Build history of the part. All positions in model axes, mm. Coordinates: 2 decimals unless noted, no trailing zeros. Order: outer loops, then holes, each group sorted by start corner. A loop starts at its lowest first (then second) coordinate and runs counter-clockwise, first axis right, second up. Notation, with made-up numbers: (51.5, 21.25) - (79.5, 21.25) arc R28 cw to (79.5, 39.25) - close; hole circle Ø1 at (5, 72). An arc over 180 degrees is marked (long way). Answer as CSV lines item,"result". Start each with the question number.
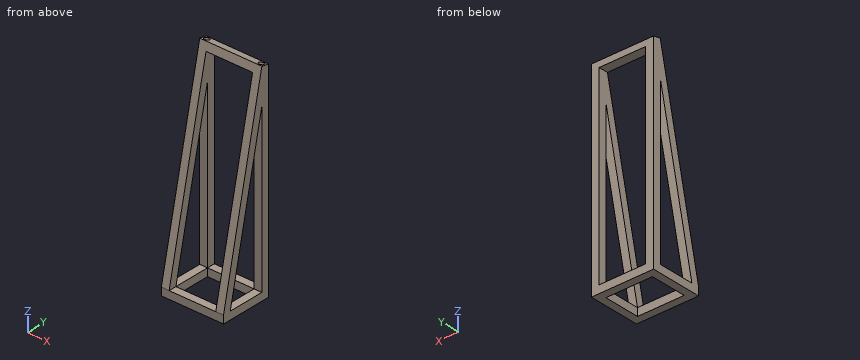
from build123d import *

# Parameters (mm, degrees)
F1_DEPTH = 30.48
F2_W     = 22.86
F2_H     = 93.98
F3_DEPTH = 25.4
F4_W     = 22.86
F4_H     = 17.78
F5_DEPTH = 25.4
F7_DEPTH = 50.8
F8_R     = 1.27
F9_DEPTH = 25.4


with BuildPart() as f1:
    # F0 (on Right) → F1 (new body)
    with BuildSketch(Plane.YZ):
        Polygon((-30.7647287846, 64.6939707769), (-52.3547287846, -33.0960292231), (-48.5447287846, -33.0960292231), (-30.7647287846, 47.4369119534), align=None)
        Polygon((-52.3547287846, -33.0960292231), (-52.3547287846, -36.9060292231), (-26.9547287846, -36.9060292231), (-26.9547287846, -33.0960292231), (-30.7647287846, -33.0960292231), (-48.5447287846, -33.0960292231), align=None)
        Polygon((-30.7647287846, -33.0960292231), (-26.9547287846, -33.0960292231), (-26.9547287846, 64.6939707769), (-30.7647287846, 47.4369119534), align=None)
        Polygon((-26.9547287846, 64.6939707769), (-30.7647287846, 64.6939707769), (-30.7647287846, 47.4369119534), align=None)
    extrude(amount=F1_DEPTH)

    # F2 (on face) → F3 (cut)
    with BuildSketch(Plane(origin=(0, -26.9547287846, 0), x_dir=(-1, 0, 0), z_dir=(0, 1, 0))):
        with Locations((-15.24, 13.8939707769)):
            Rectangle(F2_W, F2_H)
    extrude(amount=-F3_DEPTH, mode=Mode.SUBTRACT)

    # F4 (on face) → F5 (cut)
    with BuildSketch(Plane.XY.offset(-33.0960292231)):
        with Locations((15.24, -39.6547287846)):
            Rectangle(F4_W, F4_H)
    extrude(amount=-F5_DEPTH, mode=Mode.SUBTRACT)

    # F6 (on face) → F7 (cut)
    with BuildSketch(Plane(origin=(0, 0, 0), x_dir=(0, -1, 0), z_dir=(-1, 0, 0))):
        Polygon((26.9547287846, 63.8841302769), (30.7647287846, 64.6939707769), (26.9547287846, 64.6939707769), align=None)
    extrude(amount=-F7_DEPTH, mode=Mode.SUBTRACT)

    # F8 (on face) → F9 (cut)
    with BuildSketch(Plane(origin=(0, 11.8268289766, 55.640855703), x_dir=(1, 0, 0), z_dir=(0, 0.2079116908, 0.9781476007))):
        with Locations((28.575, -41.5955196646)):
            Circle(F8_R)
        with Locations((1.905, -41.5955196646)):
            Circle(F8_R)
    extrude(amount=-F9_DEPTH, mode=Mode.SUBTRACT)


solid = f1.part
(1) Band-saw the part on A-A on x = 13.5. List the corners of the cut face in (y, z), plus the area to 3 significant figures.
(2) Band-saw the part on D-D on z = 58.5. State how many separate pieces and enclosed holes the cut face has, plus the area to 3 significant figures.
(3) Drop flat-ended pins along their axis: pin 1 Ø1.9 at (x, y) = (21, -29.5) entering from +Z; pin 2 Ø1.1 at (x, y) = (16.5, -50) entering from +Z; pin 3 Ø4 at (x, z) = (26.5, -20.5) entering from -Y. Give the stop position or say it passes through.
(4) Band-saw the part on B-B on y = -36.75. List the corners of the cut face in (x, z), plus the area to 3 significant figures.
(5) Band-saw the part on C-C on z = 32.5. List the corners of the cut face in (x, y), plus the area to 3 significant figures.
(6) Probe L1, parallel to X at y = -41, z = 18; L2, parallel to X at y = -30.75, z = 52.5; L3, parallel to Y at x = 1, z = 31. List the from-to ranges inside material, lowest first. Write a range as [from, to].
Filled in:
1,outline,"(-52.35, -36.91) - (-48.54, -36.91) - (-48.54, -33.1) - (-52.35, -33.1) - close; (-31.61, 60.88) - (-26.95, 60.88) - (-26.95, 63.88) - (-30.76, 64.69) - close; (-30.76, -36.91) - (-26.95, -36.91) - (-26.95, -33.1) - (-30.76, -33.1) - close"
1,area,"43.6 mm^2"
2,separate pieces,"2"
2,enclosed holes,"2"
2,area,"29.1 mm^2"
3,pin 1,"stops at z = 64.63"
3,pin 2,"stops at z = -33.1"
3,pin 3,"stops at y = -50.01"
4,outline,"(0, -36.91) - (3.81, -36.91) - (3.81, -33.1) - (0, -33.1) - close; (0, 20.33) - (3.81, 20.33) - (3.81, 37.58) - (0, 37.58) - close; (26.67, -36.91) - (30.48, -36.91) - (30.48, -33.1) - (26.67, -33.1) - close; (26.67, 20.33) - (30.48, 20.33) - (30.48, 37.58) - (26.67, 37.58) - close"
4,area,"161 mm^2"
5,outline,"(0, -37.87) - (3.81, -37.87) - (3.81, -34.06) - (0, -34.06) - close; (0, -30.76) - (3.81, -30.76) - (3.81, -26.95) - (0, -26.95) - close; (26.67, -37.87) - (30.48, -37.87) - (30.48, -34.06) - (26.67, -34.06) - close; (26.67, -30.76) - (30.48, -30.76) - (30.48, -26.95) - (26.67, -26.95) - close"
5,area,"58.1 mm^2"
6,L1,"x = [0, 3.81], [26.67, 30.48]"
6,L2,"x = [0, 0.79], [3.02, 3.81], [26.67, 27.46], [29.69, 30.48]"
6,L3,"y = [-38.2, -34.39], [-30.76, -26.95]"
